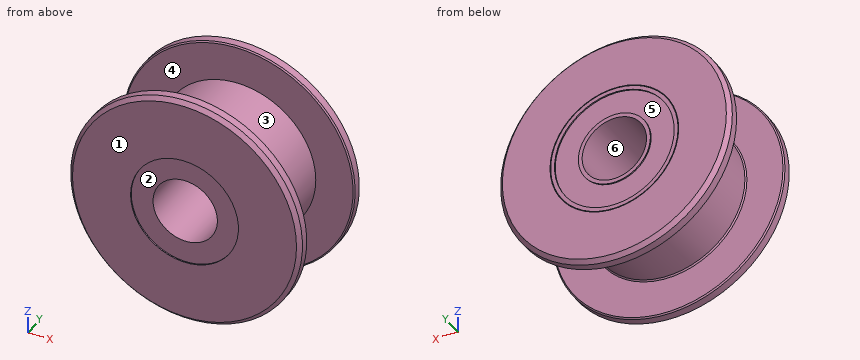
from build123d import *

# Parameters (mm, degrees)
CHAFL_N3_SIZE = 0.3
CHAFL_N4_SIZE = 0.1


with BuildPart() as part:
    # Croquis1 → Revolución3 (revolve)
    with BuildSketch(Plane.XY, mode=Mode.PRIVATE) as revoluci_n3_sk:
        Polygon((6.5, -20.750745615), (2.5, -20.750745615), (2.5, -20.850745615), (2.45, -20.850745615), (2.45, -20.750745615), (2.15, -20.750745615), (2.15, -20.850745615), (0.3, -20.850745615), (0.3, -20.750745615), (0, -20.750745615), (0, -20.850745615), (0, -29.250745615), (1.690218344, -29.250745615), (1.690218344, -29.350745615), (6.5, -29.350745615), (6.5, -28.350745615), (3.5, -28.350745615), (3.5, -21.750745615), (6.5, -21.750745615), align=None)
    revolve(revoluci_n3_sk.sketch.rotate(Axis((-2.5, -20.750745615, 0), (0, -1, 0)), 180), axis=Axis((-2.5, -20.750745615, 0), (0, -1, 0)))

    # Chaflán3
    chafl_n3_edges = [part.edges().sort_by_distance(p)[0] for p in [
        (6.5, -29.350745615, 0),
        (6.5, -20.750745615, 0),
    ]]
    chamfer(chafl_n3_edges, length=CHAFL_N3_SIZE)

    # Chaflán4
    chafl_n4_edges = [part.edges().sort_by_distance(p)[0] for p in [
        (6.5, -28.350745615, 0),
        (3.5, -28.350745615, 0),
        (6.5, -21.750745615, 0),
    ]]
    chamfer(chafl_n4_edges, length=CHAFL_N4_SIZE)


solid = part.part
Verification items for the finished model (mm, model axes). Face numbers are marked on the shaded views. A direction names the side the tool comes from. Round coordinates to 2 decimals unless told otherwise and drop trailing zeros. Loops run counter-clockwise (first coordinate to the right, second up) from the corner with the lowest first, then second, coordinate; pieces in that order, holes last. Notation, with made-up numbers: M 86,75 L 136,75 A26 ccw 136,109 Z; hole C -5,82 d2. An arc over 180 degrees is marked long. Write each question's results on one line, items separated by ' | '.
1) Gauge pin test, flat ends, axial feed: P1, Ø3, axis at x = -1, y = -25, coming from the -Z side; P2, Ø5.5, axis at x = -2.5, z = 0, coming from the -Y side; P3, Ø5, axis at x = -4.5, y = -24, coming from the -Z side. Record the tip position at first contact, or that the pin passes through.
Checks:
P1: stops at z = -6 | P2: stops at y = -29.25 | P3: stops at z = -8.93
2) Section check A-A on y = -24.25. Record the boundary of the cut face in (x, z).
Checks:
outline: C -2.5,0 d12; hole C -2.5,0 d5
3) Mould release check, pull along Z, two halves, no side actions. Record for the marked faces 1, 2 and 3: released by +Z, released by -Z, zero draft, split by the parting line, or undercut.
Checks:
face 1: zero draft | face 2: undercut | face 3: split by the parting line
4) Scan lines: L1, parallel to Y at x = 6, z = 0; L2, parallel to Z at x = -2.5, y = -24; L3, parallel to Z at x = -4.5, y = -25.5. Record each from-to range of solid material in increasing order. Write a range as from..to.
Checks:
L1: y = -29.35..-28.35, -21.75..-20.75 | L2: z = -6..-2.5, 2.5..6 | L3: z = -5.66..-1.5, 1.5..5.66
5) Access from +Z, -Z, +X, -X, +Y, -Y to the whole of each face (thin tool, end or side, straight path). Record for the marked faces 4, 5 and 6.
Checks:
face 4: none | face 5: +Y | face 6: +Y, -Y
